Model file for the job. Use its own axes, mm. Give positions to 0.01 mm unless a question says otherwise; leave off trailing zeros. Loops run counter-clockwise (first coordinate to the right, second up) from the corner with the lowest first, then second, coordinate; pieces in that order, holes last. Notation, with made-up numbers: M 44,73 L 92,73 A15 ccw 92,97 Z; hole C 71,67 d4. An arc over 180 degrees is marked long. Answer in a Markdown table with one row per item.
```python
from build123d import *

# Parameters (mm, degrees)
EXTRUDE_1_DEPTH = 2.6
SKETCH_2_W      = 0.7
SKETCH_2_H      = 0.7
EXTRUDE_2_DEPTH = 6
SKETCH_3_W      = 0.7
SKETCH_3_H      = 0.7
EXTRUDE_3_DEPTH = 3
CHAMFER_1_SIZE  = 0.2


with BuildPart() as part:
    # Sketch 1 → Extrude 1 (new body)
    with BuildSketch(Plane(origin=(0, 0, 0), x_dir=(1, 0, 0), z_dir=(0, 1, 0))):
        Polygon((-2.641860465, 1.681395349), (-2.341860465, 1.981395349), (-0.541860465, 1.981395349), (-0.241860465, 1.681395349), (-0.241860465, -0.158604651), (-0.541860465, -0.458604651), (-2.341860465, -0.458604651), (-2.641860465, -0.158604651), align=None)
    extrude(amount=EXTRUDE_1_DEPTH)

    # Sketch 2 → Extrude 2 (add)
    with BuildSketch(Plane(origin=(0, 2.6, 0), x_dir=(1, 0, 0), z_dir=(0, 1, 0))):
        with Locations((-1.441860465, 0.761395349)):
            Rectangle(SKETCH_2_W, SKETCH_2_H)
    extrude(amount=EXTRUDE_2_DEPTH)

    # Sketch 3 → Extrude 3 (add)
    with BuildSketch(Plane.XZ):
        with Locations((-1.441860465, -0.761395349)):
            Rectangle(SKETCH_3_W, SKETCH_3_H)
    extrude(amount=EXTRUDE_3_DEPTH)

    # Chamfer 1
    chamfer_1_edges = [part.edges().sort_by_distance(p)[0] for p in [
        (-1.091860465, 8.6, -0.761395349),
        (-1.441860465, 8.6, -1.111395349),
        (-1.791860465, 8.6, -0.761395349),
        (-1.441860465, 8.6, -0.411395349),
        (-1.441860465, -3, -1.111395349),
        (-1.091860465, -3, -0.761395349),
        (-1.441860465, -3, -0.411395349),
        (-1.791860465, -3, -0.761395349),
    ]]
    chamfer(chamfer_1_edges, length=CHAMFER_1_SIZE)


solid = part.part
```
(1) Saw through at D-D, the plane z = -0.2. Give the cut face in (x, y).
Established:
| item | result |
|---|---|
| outline | M -2.64,0 L -0.24,0 L -0.24,2.6 L -2.64,2.6 Z |
(2) Flat gauge pins, fed straight in: P1, Ø0.8, axis at y = 5, z = -1, coming from the +X side; P2, Ø0.6, axis at y = -2, z = -0.5, coming from the -X side; P3, Ø1, axis at x = -0.5, y = 0, coming from the -Z side; P4, Ø0.8, axis at x = -1.5, y = 4.5, coming from the -Z side. Where does each tip first touch, or does it go through?
Established:
| item | result |
|---|---|
| P1 | stops at x = -1.09 |
| P2 | stops at x = -1.79 |
| P3 | stops at z = -1.98 |
| P4 | stops at z = -1.11 |
(3) Saw through at C-C, the plane x = -0.35. Give the cut face in (y, z).
Established:
| item | result |
|---|---|
| outline | M 0,-1.79 L 2.6,-1.79 L 2.6,0.27 L 0,0.27 Z |
(4) Wall check: L1, parallel to Y at x = -2.1, z = -0.3; L2, parallel to X at y = 6.75, z = -0.5; L3, parallel to Z at x = -1.45, y = -0.5. Give the ranges that are in metal, low to high.
Established:
| item | result |
|---|---|
| L1 | y = 0 to 2.6 |
| L2 | x = -1.79 to -1.09 |
| L3 | z = -1.11 to -0.41 |
(5) Saw through at B-B, the plane y = 0.25. Give the cut face in (x, z).
Established:
| item | result |
|---|---|
| outline | M -2.64,-1.68 L -2.34,-1.98 L -0.54,-1.98 L -0.24,-1.68 L -0.24,0.16 L -0.54,0.46 L -2.34,0.46 L -2.64,0.16 Z |
(6) Saw through at A-A, the plane z = -0.8. Give the cut face in (x, y).
Established:
| item | result |
|---|---|
| outline | M -2.64,0 L -1.79,0 L -1.79,-2.8 L -1.59,-3 L -1.29,-3 L -1.09,-2.8 L -1.09,0 L -0.24,0 L -0.24,2.6 L -1.09,2.6 L -1.09,8.4 L -1.29,8.6 L -1.59,8.6 L -1.79,8.4 L -1.79,2.6 L -2.64,2.6 Z |
